Design review of the part built by this model. Coordinates are the model's own, in mm. A direction names the side the tool comes from. Give positions to 0.01 mm unless a question says otherwise; leave off trailing zeros. Write each loop counter-clockwise with the first axis right and the second up, starting at its lowest first coordinate (ties: lowest second). Pieces come first, ordered by that corner, then holes. Notation, with made-up numbers: (65.5, 10) -> (123.5, 10) arc R29 ccw to (123.5, 37) -> close; hole circle Ø2 at (16.25, 37.5). An arc over 180 degrees is marked (long way). Write each question's results on one line, items separated by ' | '. Start each with the question number.
(1) Take a section at D-D (y = 9.25). State the section outline as (x, z) points, plus the area to 3 significant figures.
(2) Take a section at C-C (x = -40). State the section outline as (y, z) points, plus the area to 3 significant figures.
(3) Clearance check with flat-ended pins moving along their axes: pin 1 (4 mm diameter, centred on x = 15.5, z = -4.5, fed in from -Y); pin 2 (14 mm diameter, centred on x = 40, z = 40, fed in from -Y); pin 3 (4 mm diameter, centred on y = -3.5, z = 7.5, fed in from -X); pin 4 (2.5 mm diameter, centred on x = -8.5, y = -1.5, fed in from -Z). State where each tip first meets the part, or that it passes through.
(4) Take a section at B-B (z = -40). State the section outline as (x, y) points.
(5) Mouldability with a two-part tool opening along X and no side actions: class faces 1 (the face through (-1, -2, 50)), 2 (the face through (50, -2, -1)), 3 (the face through (1.32, -2.54, 29.97)) as released by +X, released by -X, zero draft, split by the parting line, or undercut.
(6) To check wall thickness, follow probe 1 along X at (y, z) = (14.25, -40); probe 2 along X at (y, z) = (0.3, 0); probe 3 along Y at (x, z) = (-11, 33). State the ranges of each line that lie inside material, in increasing order.
(7) For faces 4 (the face through (48, -3, 49)), 5 (the face through (24, 19, -13)), 6 (the face through (-1, -2, -50)), 7 (the face through (-18, 21, 0)), list the 3-axis set-ups (+Z, -Z, +X, -X, +Y, -Y) from which the entire face can be reached by the end or side of a thin tool; tool diameter is ignored.
from build123d import *

# Parameters (mm, degrees)
SKETCH_1_W          = 112
SKETCH_1_H          = 112
EXTRUDE_1_DEPTH     = 19
SKETCH_2_R          = 25.75
EXTRUDE_2_DEPTH     = 5
SKETCH_3_W          = 100
SKETCH_3_H          = 100
EXTRUDE_3_DEPTH     = 5
SKETCH_4_R          = 30
CUT_EXTRUDE_1_DEPTH = 5
SKETCH_5_R          = 26
CUT_EXTRUDE_2_DEPTH = 1
SKETCH_6_R          = 21
CUT_EXTRUDE_3_DEPTH = 20
SKETCH_7_R          = 17.5
CUT_EXTRUDE_4_DEPTH = 85.338603261
SKETCH_8_R          = 7.9
CUT_EXTRUDE_5_DEPTH = 83.752643462
FILLET_1_R          = 5
FILLET_2_R          = 1


with BuildPart() as part:
    # 草图1 → 凸台-拉伸1 (new body)
    with BuildSketch(Plane(origin=(0, 0, 0), x_dir=(1, 0, 0), z_dir=(0, 1, 0))):
        Rectangle(SKETCH_1_W, SKETCH_1_H)
    extrude(amount=EXTRUDE_1_DEPTH)

    # 草图2 → 凸台-拉伸2 (add)
    with BuildSketch(Plane(origin=(0, 19, 0), x_dir=(1, 0, 0), z_dir=(0, 1, 0))):
        with Locations(Location((0, 0, 0), (0, 0, 270))):
            Circle(SKETCH_2_R)
    extrude(amount=EXTRUDE_2_DEPTH)

    # 草图3 → 凸台-拉伸3 (add)
    with BuildSketch(Plane.XZ):
        Rectangle(SKETCH_3_W, SKETCH_3_H)
    extrude(amount=EXTRUDE_3_DEPTH)

    # 草图4 → 切除-拉伸1 (cut)
    with BuildSketch(Plane.XZ.offset(5)):
        with Locations(Location((0, 0, 0), (0, 0, 270))):
            Circle(SKETCH_4_R)
    extrude(amount=-CUT_EXTRUDE_1_DEPTH, mode=Mode.SUBTRACT)

    # 草图5 → 切除-拉伸2 (cut)
    with BuildSketch(Plane.XZ):
        with Locations(Location((0, 0, 0), (0, 0, 270))):
            Circle(SKETCH_5_R)
    extrude(amount=-CUT_EXTRUDE_2_DEPTH, mode=Mode.SUBTRACT)

    # 草图6 → 切除-拉伸3 (cut)
    with BuildSketch(Plane.XZ.offset(-1)):
        with Locations(Location((0, 0, 0), (0, 0, 270))):
            Circle(SKETCH_6_R)
    extrude(amount=-CUT_EXTRUDE_3_DEPTH, mode=Mode.SUBTRACT)

    # 草图7 → 切除-拉伸4 (cut, through all)
    with BuildSketch(Plane(origin=(0, 24, 0), x_dir=(1, 0, 0), z_dir=(0, 1, 0))):
        with Locations(Location((0, 0, 0), (0, 0, 270))):
            Circle(SKETCH_7_R)
    extrude(amount=-CUT_EXTRUDE_4_DEPTH, mode=Mode.SUBTRACT)

    # 草图8 → 切除-拉伸5 (cut, through all)
    with BuildSketch(Plane(origin=(0, 19, 0), x_dir=(1, 0, 0), z_dir=(0, 1, 0))):
        with Locations(Location((-40, 40, 0), (0, 0, 270))):
            Circle(SKETCH_8_R)
        with Locations(Location((40, 40, 0), (0, 0, 270))):
            Circle(SKETCH_8_R)
        with Locations(Location((40, -40, 0), (0, 0, 270))):
            Circle(SKETCH_8_R)
        with Locations(Location((-40, -40, 0), (0, 0, 270))):
            Circle(SKETCH_8_R)
    extrude(amount=-CUT_EXTRUDE_5_DEPTH, mode=Mode.SUBTRACT)

    # 圆角1
    fillet_1_edges = [part.edges().sort_by_distance(p)[0] for p in [
        (50, -2.5, -50),
        (50, -2.5, 50),
        (-50, -2.5, 50),
        (-50, -2.5, -50),
        (56, 9.5, 56),
        (-56, 9.5, 56),
        (-56, 9.5, -56),
        (56, 9.5, -56),
    ]]
    fillet(fillet_1_edges, radius=FILLET_1_R)

    # 圆角2
    fillet_2_edges = [part.edges().sort_by_distance(p)[0] for p in [
        (0, 21, 21),
    ]]
    fillet(fillet_2_edges, radius=FILLET_2_R)


solid = part.part
Report:
1) outline: (-56, -51) arc R5 ccw to (-51, -56) -> (51, -56) arc R5 ccw to (56, -51) -> (56, 51) arc R5 ccw to (51, 56) -> (-51, 56) arc R5 ccw to (-56, 51) -> close; hole circle Ø15.8 at (-40, -40); hole circle Ø15.8 at (-40, 40); hole circle Ø42 at (0, 0); hole circle Ø15.8 at (40, -40); hole circle Ø15.8 at (40, 40) | area: 10,400 mm2
2) outline: (-5, -50) -> (0, -50) -> (0, -56) -> (19, -56) -> (19, -47.9) -> (-5, -47.9) -> close; (-5, -32.1) -> (19, -32.1) -> (19, 32.1) -> (-5, 32.1) -> close; (-5, 47.9) -> (19, 47.9) -> (19, 56) -> (0, 56) -> (0, 50) -> (-5, 50) -> close | area: 1,870 mm2
3) pin 1: y = 21 | pin 2: through | pin 3: x = -50 | pin 4: z = -50
4) outline: (-56, 0) -> (-50, 0) -> (-50, -5) -> (-47.9, -5) -> (-47.9, 19) -> (-56, 19) -> close; (-32.1, -5) -> (32.1, -5) -> (32.1, 19) -> (-32.1, 19) -> close; (47.9, -5) -> (50, -5) -> (50, 0) -> (56, 0) -> (56, 19) -> (47.9, 19) -> close
5) face 1: zero draft | face 2: released by +X | face 3: undercut
6) probe 1: -56 to -47.9, -32.1 to 32.1, 47.9 to 56 | probe 2: -56 to -26, 26 to 56 | probe 3: -5 to 19
7) face 4: +Z, +X, -Y | face 5: +Y | face 6: -Z, +X, -X, -Y | face 7: -Y
